Verification items for the finished model (mm, model axes). Round coordinates to 2 decimals unless told otherwise and drop trailing zeros. Order: outer loops, then holes, each group sorted by start corner. A loop starts at its lowest first (then second) coordinate and runs counter-clockwise, first axis right, second up. Notation, with made-up numbers: (62, 32.5) -> (82, 32.5) arc R6 cw to (82, 43.5) -> close; hole circle Ø7 at (-31.75, 58.5). An arc over 180 degrees is marked (long way). Return JSON: item names as keys, results as strings. Group by question number.
Item 1: Scan lines: probe 1 along Y at (x, z) = (1.45, -5); probe 2 along Z at (x, y) = (0.8, 14); probe 3 along Z at (x, y) = (0.2, 56.5). Record each from-to range of solid material in increasing order. Write a range as from..to.
Item 2: Sectioned sample at B-B on y = 5. Record the cut outline in (x, z).
Item 3: Sectioned sample at A-A on z = -65. Record the cut outline in (x, y).
Item 4: Depth check by flat-ended pin: pin 1 Ø3.5 at (y, z) = (65, -5) entering from +X; pin 2 Ø2.5 at (y, z) = (56.92, -56.61) entering from -X. Enter the tip coordinate at first touch or a pass-through.
Autodesk Inventor part; units mm, degrees
ref_plane "YZ Plane" through (0, 0, 0) normal (1, 0, 0) x (0, 1, 0)
ref_plane "XZ Plane" through (0, 0, 0) normal (0, 1, 0) x (-1, 0, 0)
ref_plane "XY Plane" through (0, 0, 0) normal (0, 0, 1) x (1, 0, 0)
sketch "Sketch1" plane through (0, 0, 0) normal (1, 0, 0) x (0, 1, 0)
  line L0 (8.5457, 136.9798) -> (8.5457, 103.4797)
  spline S0 degree 3 poles (19.375, 147.8091) (18.6641, 147.8091) (17.9599, 147.7397) (17.2623, 147.601) (16.5652, 147.4624) (15.8881, 147.2569) (15.2308, 146.9847) (14.5742, 146.7128) (13.9501, 146.3792) (13.3586, 145.984) (12.7676, 145.5892) (12.2206, 145.1402) (11.7175, 144.6372) (11.215, 144.1347) (10.766, 143.5877) (10.3708, 142.9962) (9.9759, 142.4053) (9.6423, 141.7812) (9.37, 141.1239) (9.098, 140.4674) (8.8926, 139.7902) (8.7538, 139.0925) (8.6151, 138.3952) (8.5457, 137.691) (8.5457, 136.9798) knots 0 0 0 0 0.125 0.125 0.125 0.25 0.25 0.25 0.375 0.375 0.375 0.5 0.5 0.5 0.625 0.625 0.625 0.75 0.75 0.75 0.875 0.875 0.875 1 1 1 1
  line L1 (52.875, 147.8091) -> (19.375, 147.8091)
  arc A0 (58.801, 146.0438) -> (54.8456, 147.6282) centre (52.875, 136.9798) ccw
  ellipse E0 centre (52.881, 136.9737) end of major axis (52.8771, 126.1401) minor radius 10.825 (61.939, 142.9057) -> (58.801, 146.0438) ccw
  line L2 (63.7043, 103.4798) -> (63.7043, 136.9798)
  spline S1 degree 3 poles (58.801, 94.4157) (59.4265, 94.8247) (60.0037, 95.2936) (60.5324, 95.8223) (61.061, 96.3507) (61.5298, 96.9279) (61.939, 97.5537) knots 0 0 0 0 0.5 0.5 0.5 1 1 1 1
  spline S2 degree 3 poles (52.875, 92.6505) (53.5374, 92.6505) (54.1943, 92.7107) (54.8456, 92.8313) knots 0 0 0 0 1 1 1 1
  line L3 (19.375, 92.6505) -> (52.875, 92.6505)
  spline S3 degree 3 poles (10.311, 97.5538) (10.72, 96.9282) (11.1888, 96.3511) (11.7175, 95.8223) (12.246, 95.2938) (12.8231, 94.825) (13.449, 94.4158) knots 0 0 0 0 0.5 0.5 0.5 1 1 1 1
  arc A1 (57.625, 140.4108) -> (57.625, 143.0488) centre (57.625, 141.7298) ccw
  arc A2 (57.625, 143.0488) -> (57.625, 140.4108) centre (57.625, 141.7298) ccw
  arc A3 (57.625, 97.4108) -> (57.625, 100.0488) centre (57.625, 98.7298) ccw
  arc A4 (57.625, 100.0488) -> (57.625, 97.4108) centre (57.625, 98.7298) ccw
  arc A5 (14.625, 97.4108) -> (14.625, 100.0488) centre (14.625, 98.7298) ccw
  arc A6 (14.625, 100.0488) -> (14.625, 97.4108) centre (14.625, 98.7298) ccw
  circle A7 centre (14.625, 141.7298) radius 1.319
  arc A8 (63.5235, 138.9504) -> (61.939, 142.9057) centre (52.875, 136.9798) ccw
  line L4 (0, 0) -> (70, 0)
  line L5 (70, 0) -> (70, -70)
  line L6 (70, -70) -> (0, -70)
  line L7 (0, -70) -> (0, 0)
  point P0 (36.125, 120.2298)
  point P1 (63.5235, 101.5091)
  point P2 (62.9439, 99.4934)
  point P3 (56.8613, 93.4109)
  point P4 (57.625, 142.7363)
  dimension "d0" = 70
  dimension "d1" = 70
extrude "Extrusion1" add sketch "Sketch1" along normal blind 3 contours L4 L5 L6 L7
sketch "Sketch2" plane through (3, 0, 0) normal (1, 0, 0) x (0, 0, -1)
  line L0 (7.5282, 52.1652) -> (7.5282, 18.6652)
  spline S0 degree 3 poles (18.3575, 62.9945) (17.6466, 62.9945) (16.9424, 62.9251) (16.2448, 62.7864) (15.5477, 62.6478) (14.8706, 62.4424) (14.2133, 62.1702) (13.5567, 61.8982) (12.9326, 61.5646) (12.341, 61.1694) (11.7501, 60.7746) (11.2031, 60.3257) (10.7, 59.8227) (10.1975, 59.3201) (9.7485, 58.7731) (9.3533, 58.1816) (8.9584, 57.5907) (8.6248, 56.9666) (8.3525, 56.3094) (8.0805, 55.6528) (7.8751, 54.9756) (7.7363, 54.2779) (7.5976, 53.5807) (7.5282, 52.8764) (7.5282, 52.1652) knots 0 0 0 0 0.125 0.125 0.125 0.25 0.25 0.25 0.375 0.375 0.375 0.5 0.5 0.5 0.625 0.625 0.625 0.75 0.75 0.75 0.875 0.875 0.875 1 1 1 1
  line L1 (51.8575, 62.9945) -> (18.3575, 62.9945)
  arc A0 (57.7835, 61.2292) -> (53.8281, 62.8137) centre (51.8575, 52.1652) ccw
  ellipse E0 centre (51.8635, 52.1592) end of major axis (51.8596, 41.3255) minor radius 10.825 (60.9215, 58.0912) -> (57.7835, 61.2292) ccw
  line L2 (62.6868, 18.6652) -> (62.6868, 52.1652)
  spline S1 degree 3 poles (57.7835, 9.6012) (58.409, 10.0102) (58.9862, 10.479) (59.5149, 11.0077) (60.0434, 11.5362) (60.5123, 12.1133) (60.9215, 12.7392) knots 0 0 0 0 0.5 0.5 0.5 1 1 1 1
  spline S2 degree 3 poles (51.8575, 7.8359) (52.5199, 7.8359) (53.1768, 7.8962) (53.8281, 8.0167) knots 0 0 0 0 1 1 1 1
  line L3 (18.3575, 7.8359) -> (51.8575, 7.8359)
  spline S3 degree 3 poles (9.2935, 12.7392) (9.7025, 12.1137) (10.1713, 11.5365) (10.7, 11.0077) (11.2285, 10.4792) (11.8056, 10.0104) (12.4315, 9.6012) knots 0 0 0 0 0.5 0.5 0.5 1 1 1 1
  arc A1 (56.6075, 55.5962) -> (56.6075, 58.2342) centre (56.6075, 56.9152) ccw
  arc A2 (56.6075, 58.2342) -> (56.6075, 55.5962) centre (56.6075, 56.9152) ccw
  arc A3 (56.6075, 12.5962) -> (56.6075, 15.2342) centre (56.6075, 13.9152) ccw
  arc A4 (56.6075, 15.2342) -> (56.6075, 12.5962) centre (56.6075, 13.9152) ccw
  arc A5 (13.6075, 12.5962) -> (13.6075, 15.2342) centre (13.6075, 13.9152) ccw
  arc A6 (13.6075, 15.2342) -> (13.6075, 12.5962) centre (13.6075, 13.9152) ccw
  circle A7 centre (13.6075, 56.9152) radius 1.319
  arc A8 (62.506, 54.1358) -> (60.9215, 58.0912) centre (51.8575, 52.1652) ccw
  point P0 (0, 0)
  point P1 (35.1075, 35.4152)
  point P2 (62.506, 16.6946)
  point P3 (61.9264, 14.6789)
  point P4 (55.8438, 8.5963)
  point P5 (56.6075, 57.9217)
extrude "Extrusion2" cut sketch "Sketch2" against normal blind 68.4375
sketch "Sketch3" plane through (3, 0, 0) normal (1, 0, 0) x (0, 0, -1)
  circle A0 centre (5, 5) radius 1.5
  circle A1 centre (5, 65) radius 1.5
  circle A2 centre (65, 65) radius 1.5
  circle A3 centre (65, 5) radius 1.5
  point P0 (0, 0)
  dimension "d6" = 3
  dimension "d7" = 3
  dimension "d8" = 3
  dimension "d9" = 3
extrude "Extrusion3" cut sketch "Sketch3" against normal blind 39.5125
equation "\"BendRadius\" = Thickness"
equation "\"BendReliefWidth\" = Thickness"
equation "\"BendReliefDepth\" = 0.5 * Thickness"
equation "\"CornerReliefSize\" = 4 * Thickness"
equation "\"MinimumRemnant\" = 2 * Thickness"
equation "\"TransitionRadius\" = BendRadius"
equation "\"JacobiRadiusSize\" = BendRadius"
equation "\"GapSize\" = Thickness"
properties part number "lidar_plate" material "Aluminum 6061"
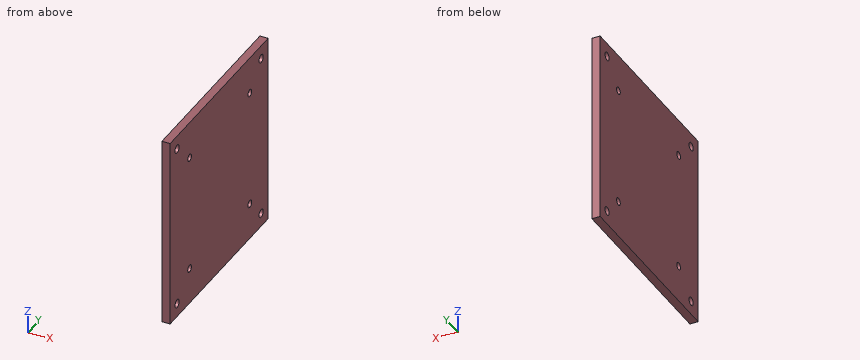
Recorded:
{
 "1": {"probe 1": "0..3.5, 6.5..63.5, 66.5..70", "probe 2": "-70..-57.92, -55.29..-14.92, -12.29..0", "probe 3": "-70..-57.86, -55.36..-14.86, -12.36..0"},
 "2": {"outline": "(0, -70) -> (3, -70) -> (3, -66.5) -> (0, -66.5) -> close; (0, -63.5) -> (3, -63.5) -> (3, -6.5) -> (0, -6.5) -> close; (0, -3.5) -> (3, -3.5) -> (3, 0) -> (0, 0) -> close"},
 "3": {"outline": "(0, 0) -> (3, 0) -> (3, 3.5) -> (0, 3.5) -> close; (0, 6.5) -> (3, 6.5) -> (3, 63.5) -> (0, 63.5) -> close; (0, 66.5) -> (3, 66.5) -> (3, 70) -> (0, 70) -> close"},
 "4": {"pin 1": "x = 3", "pin 2": "through"}
}
